The model under review builds one solid part; all positions refer to its coordinate system, in mm. A direction names the side the tool comes from. Coordinates: 2 decimals unless noted, no trailing zeros. Write each loop counter-clockwise with the first axis right and the second up, starting at its lowest first coordinate (ties: lowest second). Pieces come first, ordered by that corner, then holes. Notation, with made-up numbers: (87.25, 31.5) - (131.25, 31.5) arc R32 cw to (131.25, 61.5) - close; hole circle Ø7 at (-33.75, 59). An arc over 180 degrees is marked (long way). Put each result on its own line as item: value.
from build123d import *

# Parameters (mm, degrees)
SKETCH1_R           = 75
BOSS_EXTRUDE1_DEPTH = 14
SKETCH2_R           = 13
CUT_EXTRUDE1_DEPTH  = 8
SKETCH3_R           = 12
CUT_EXTRUDE2_DEPTH  = 8
SKETCH4_R           = 5
CUT_EXTRUDE4_DEPTH  = 107.98598039
SKETCH5_R           = 1.75
CUT_EXTRUDE5_DEPTH  = 107.98598039


with BuildPart() as part:
    # Sketch1 → Boss-Extrude1 (new body)
    with BuildSketch(Plane(origin=(0, 0, 0), x_dir=(1, 0, 0), z_dir=(0, 1, 0))):
        with Locations(Location((0, 0, 0), (0, 0, 270))):
            Circle(SKETCH1_R)
    extrude(amount=BOSS_EXTRUDE1_DEPTH)

    # Sketch2 → Cut-Extrude1 (cut)
    with BuildSketch(Plane(origin=(0, 14, 0), x_dir=(1, 0, 0), z_dir=(0, 1, 0))):
        with Locations(Location((0, 0, 0), (0, 0, 270))):
            Circle(SKETCH2_R)
    extrude(amount=-CUT_EXTRUDE1_DEPTH, mode=Mode.SUBTRACT)

    # Sketch3 → Cut-Extrude2 (cut)
    with BuildSketch(Plane(origin=(0, 6, 0), x_dir=(1, 0, 0), z_dir=(0, 1, 0))):
        with Locations(Location((0, 0, 0), (0, 0, 270))):
            Circle(SKETCH3_R)
    extrude(amount=-CUT_EXTRUDE2_DEPTH, mode=Mode.SUBTRACT)

    # Sketch4 → Cut-Extrude4 (cut, through all)
    with BuildSketch(Plane(origin=(0, 14, 0), x_dir=(1, 0, 0), z_dir=(0, 1, 0))):
        with Locations(Location((0, 62.5, 0), (0, 0, 270))):
            Circle(SKETCH4_R)
        with Locations(Location((-54.126587737, -31.25, 0), (0, 0, 270))):
            Circle(SKETCH4_R)
        with Locations(Location((54.126587737, -31.25, 0), (0, 0, 270))):
            Circle(SKETCH4_R)
    extrude(amount=-CUT_EXTRUDE4_DEPTH, mode=Mode.SUBTRACT)

    # Sketch5 → Cut-Extrude5 (cut, through all)
    with BuildSketch(Plane(origin=(0, 14, 0), x_dir=(1, 0, 0), z_dir=(0, 1, 0))):
        with Locations(Location((-15.201634245, -47.250661584, 0), (0, 0, 270))):
            Circle(SKETCH5_R)
        with Locations(Location((10.798365755, -47.250661584, 0), (0, 0, 270))):
            Circle(SKETCH5_R)
    extrude(amount=-CUT_EXTRUDE5_DEPTH, mode=Mode.SUBTRACT)


solid = part.part
1. For pin 1 Ø13 at (x, z) = (-1, -2) entering from +Y; pin 2 Ø4 at (y, z) = (3.5, -52) entering from +X; pin 3 Ø1.5 at (x, z) = (21.5, 23.5) entering from -Y; pin 4 Ø3 at (x, y) = (19, 4) entering from +Z, all flat-tipped, find the tip position at first contact; note any pin that passes through.
Determined:
pin 1: passes through
pin 2: stops at x = 55.9
pin 3: stops at y = 0
pin 4: stops at z = 72.93
2. Consider section C-C on y = 4.25. State the section outline as (x, z) points, plus the area to 3 significant figures.
Determined:
outline: circle Ø150 at (0, 0); hole circle Ø10 at (-54.13, 31.25); hole circle Ø3.5 at (-15.2, 47.25); hole circle Ø24 at (0, 0); hole circle Ø10 at (0, -62.5); hole circle Ø3.5 at (10.8, 47.25); hole circle Ø10 at (54.13, 31.25)
area: 17,000 mm^2
3. Consider section D-D on z = 29.5. State the section outline as (x, y) points.
Determined:
outline: (-68.95, 0) - (-58.81, 0) - (-58.81, 14) - (-68.95, 14) - close; (-49.44, 0) - (49.44, 0) - (49.44, 14) - (-49.44, 14) - close; (58.81, 0) - (68.95, 0) - (68.95, 14) - (58.81, 14) - close
4. To check wall thickness, follow probe 1 along X at (y, z) = (12, 46.5); probe 2 along X at (y, z) = (10.25, 0); probe 3 along Z at (x, y) = (3, 3). State the ranges of each line that lie inside material, in increasing order.
Determined:
probe 1: x = -58.85 to -16.78, -13.62 to 9.22, 12.38 to 58.85
probe 2: x = -75 to -13, 13 to 75
probe 3: z = -74.94 to -66.5, -58.5 to -11.62, 11.62 to 74.94
5. Consider section B-B on z = 0. State the section outline as (x, y) points.
Determined:
outline: (-75, 0) - (-12, 0) - (-12, 6) - (-13, 6) - (-13, 14) - (-75, 14) - close; (12, 0) - (75, 0) - (75, 14) - (13, 14) - (13, 6) - (12, 6) - close
6. The part is to be moulded in two halves that separate along Z. For faces 1 (the cylindrical face through (3.604, 3.042, 11.446)), 2 (the cylindrical face through (-45.636, 6.902, -59.517)), 3 (the flat face through (-16, 14, -1)), say which applies: +Z half, -Z half, draft (parallel to the pull), parting line (faces both ways), or undercut.
Determined:
face 1: undercut
face 2: parting line
face 3: draft
7. Machinability: for faces 4 (the cylindrical face through (-7.91, 10.056, -10.316)), 5 (the flat face through (-16, 0, -1)), which of the approach directions +Z, -Z, +X, -X, +Y, -Y give a long, thin tool a straight path to every point of the face, cutting with its end or side? Answer none if there is none.
Determined:
face 4: +Y
face 5: +Z, -Z, +X, -X, -Y
8. Consider section A-A on x = 0. State the section outline as (y, z) points.
Determined:
outline: (0, -75) - (14, -75) - (14, -67.5) - (0, -67.5) - close; (0, -57.5) - (14, -57.5) - (14, -13) - (6, -13) - (6, -12) - (0, -12) - close; (0, 12) - (6, 12) - (6, 13) - (14, 13) - (14, 75) - (0, 75) - close
